Here's how the part is built. I have some questions about the finished solid (model axes, mm). A direction names the side the tool comes from. Give positions to 0.01 mm unless a question says otherwise; leave off trailing zeros. Write each loop counter-clockwise with the first axis right and the second up, starting at its lowest first coordinate (ties: lowest second). Pieces come first, ordered by that corner, then holes. Notation, with made-up numbers: (45, 59.25) - (76, 59.25) arc R10 ccw to (76, 76.25) - close; hole circle Ø11 at (79, -0.75). An arc over 180 degrees is marked (long way). One line per item, written item: value. Start each with the question number.
1) I'm going to push a flat-ended pin straight in: P1, Ø3, axis at x = 70.5, y = -22.5, coming from the +Z side. Where does the tip first touch, or does it pass through?
2) On a 3-axis mill with a long thin cutter (end or side, diameter ignored), from which of +Z, -Z, +X, -X, +Y, -Y can I reach the whole of each face in a straight line? I mean faces 1 (the flat face through (86, -1, 53)), 2 (the flat face through (174.5, -109.5, 45)), 3 (the flat face through (86.28, -8.96, 8.72)). Say none if no direction works.
3) Imagine slicing it at C-C on z = 37.5. Write out the boundary of the cut face in (x, y).
4) Imagine slicing it at A-A on y = -38.5. Write out the boundary of the cut face in (x, z).
5) Imagine slicing it at B-B on z = 54. Write out the boundary of the cut face in (x, y).
6) Please list where these lines run through material, in increasing order: L1, parallel to Y at x = 91, z = 55; L2, parallel to X at y = -134.5, z = 26; L3, parallel to Z at x = 143, y = -78. Write a range as [from, to].
7) We'd pull the mould along X, two halves only. Please class faces 4 (the flat face through (86, 0, 52)), 5 (the flat face through (175, -90, 35)), 6 (the flat face through (86, -88, 1)): +X half, -X half, draft (parallel to the pull), parting line (faces both ways), or undercut.
8) Imagine slicing it at D-D on x = 116.5. Write out the boundary of the cut face in (y, z).
from build123d import *

# Parameters (mm, degrees)
F0_W        = 175
F0_H        = 178
F1_DEPTH    = 88
F2_SIZE     = 17.678
F3_T        = -1
F4_W        = 45
F4_H        = 25
F5_DEPTH    = 2
F6_T1_DEPTH = 1
F7_SIZE     = 4


# Not quite as in the source:
# - a fillet or chamfer that OpenCascade refuses, or shapes differently, is made with other operations: its cross-section is extruded or revolved along the edge and cut away or added


with BuildPart() as f1:
    # F0 (on Top) → F1 (new body)
    with BuildSketch(Plane.XY):
        with Locations((87.5, -89)):
            Rectangle(F0_W, F0_H)
    extrude(amount=F1_DEPTH)

    # F2
    f2_edges = [f1.edges().sort_by_distance(p)[0] for p in [
        (87.5, -178, 0),
        (87.5, 0, 0),
    ]]
    chamfer(f2_edges, length=F2_SIZE)

    # F3
    f3_openings = [f1.faces().sort_by_distance(p)[0] for p in [
        (87.5, -89, 88),
    ]]
    offset(amount=F3_T, openings=f3_openings)

    # F4 (on face) → F5 (cut)
    with BuildSketch(Plane.YZ.offset(175)):
        with Locations((-89, 55.5)):
            Rectangle(F4_W, F4_H)
    extrude(amount=-F5_DEPTH, mode=Mode.SUBTRACT)

    # F6: chamfer of 4 x 22.6851272785 on 2 edges, made by hand

    # F6_s2 → F6_t1 (join)
    with BuildSketch(Plane.YZ.offset(174)):
        Polygon((-111.5, 64), (-88.8148727215, 68), (-111.5, 68), align=None)
        Polygon((-66.5, 64), (-89.1851272785, 68), (-66.5, 68), align=None)
    extrude(amount=F6_T1_DEPTH)

    # F7
    f7_edges = [f1.edges().sort_by_distance(p)[0] for p in [
        (174.5, -111.5, 43),
        (174.5, -66.5, 43),
    ]]
    chamfer(f7_edges, length=F7_SIZE)


solid = f1.part
Numbers:
1. P1: z = 1
2. face 1: +Z
2. face 2: +X
2. face 3: -Z, +X, -X, +Y
3. outline: (0, -178) - (175, -178) - (175, 0) - (0, 0) - close; hole (1, -177) - (174, -177) - (174, -1) - (1, -1) - close
4. outline: (0, 0) - (175, 0) - (175, 88) - (174, 88) - (174, 1) - (1, 1) - (1, 88) - (0, 88) - close
5. outline: (0, -178) - (175, -178) - (175, -111.5) - (174, -111.5) - (174, -177) - (1, -177) - (1, -1) - (174, -1) - (174, -66.5) - (175, -66.5) - (175, 0) - (0, 0) - close
6. L1: [-178, -177], [-1, 0]
6. L2: [0, 1], [174, 175]
6. L3: [0, 1]
7. face 4: draft
7. face 5: +X half
7. face 6: undercut
8. outline: (-178, 17.68) - (-160.32, 0) - (-17.68, 0) - (0, 17.68) - (0, 88) - (-1, 88) - (-1, 18.09) - (-18.09, 1) - (-159.91, 1) - (-177, 18.09) - (-177, 88) - (-178, 88) - close
